```python
from build123d import *

# Parameters (mm, degrees)
SKETCH1_R           = 1.5
BOSS_EXTRUDE1_DEPTH = 5


with BuildPart() as part:
    # Sketch1 → Boss-Extrude1 (new body)
    with BuildSketch(Plane.XY):
        with BuildLine():
            Line((75.000000208, -15), (-75.000000208, -15))
            Line((-75.000000208, -15), (-75.000000208, 15))
            Line((-75.000000208, 15), (75.000000208, 15))
            ThreePointArc((75.000000208, 15), (89.999999792, 0), (75.000000208, -15))
        make_face()
        with Locations((75, 7)):
            Circle(SKETCH1_R, mode=Mode.SUBTRACT)
        with Locations((82, 0)):
            Circle(SKETCH1_R, mode=Mode.SUBTRACT)
        with Locations(Location((68, 0, 0), (0, 0, 180))):
            Circle(SKETCH1_R, mode=Mode.SUBTRACT)
        with Locations(Location((75, -7, 0), (0, 0, 180))):
            Circle(SKETCH1_R, mode=Mode.SUBTRACT)
        with Locations((-63.000000208, 0)):
            Circle(SKETCH1_R, mode=Mode.SUBTRACT)
        with Locations((-63.000000208, 10)):
            Circle(SKETCH1_R, mode=Mode.SUBTRACT)
        with Locations((-63.000000208, -10)):
            Circle(SKETCH1_R, mode=Mode.SUBTRACT)
    extrude(amount=BOSS_EXTRUDE1_DEPTH)


solid = part.part
```
Model file for the job. Use its own axes, mm. Give positions to 0.01 mm unless a question says otherwise; leave off trailing zeros. Loops run counter-clockwise (first coordinate to the right, second up) from the corner with the lowest first, then second, coordinate; pieces in that order, holes last. Notation, with made-up numbers: (47.25, 22.25) - (65.25, 22.25) arc R8 ccw to (65.25, 36.25) - close; hole circle Ø4 at (6.5, 63.5). An arc over 180 degrees is marked (long way). One line per item, written item: value. Start each with the question number.
1. Slice it at A-A (y = 0). List the corners of the cut face in (x, z).
2. Slice it at B-B (z = 1.55). List the corners of the cut face in (x, y).
3. Slice it at D-D (x = -63). List the corners of the cut face in (y, z).
4. Slice it at C-C (x = 68). List the corners of the cut face in (y, z).
5. Pull direction Y, two halves, no side cores. Call faces 1 (the flat face through (-1, 15, 2)), 2 (the cylindrical face through (-64.2, 9.1, 2.5)), 3 (the flat face through (9, 0, 5)): pulls with the +Y half, pulls with the -Y half, needs draft (parallel to the pull), parting line crosses it, or undercut.
6. Probe L1, parallel to Y at x = -63, z = 2.3; L2, parallel to X at y = 9, z = 1.5; L3, parallel to Y at x = 82, z = 4. List the from-to ranges inside material, lowest first. Write a range as from..to.
Solution:
1. outline: (-75, 0) - (-64.5, 0) - (-64.5, 5) - (-75, 5) - close; (-61.5, 0) - (66.5, 0) - (66.5, 5) - (-61.5, 5) - close; (69.5, 0) - (80.5, 0) - (80.5, 5) - (69.5, 5) - close; (83.5, 0) - (90, 0) - (90, 5) - (83.5, 5) - close
2. outline: (-75, -15) - (75, -15) arc R15 ccw to (75, 15) - (-75, 15) - close; hole circle Ø3 at (-63, -10); hole circle Ø3 at (-63, 0); hole circle Ø3 at (-63, 10); hole circle Ø3 at (68, 0); hole circle Ø3 at (75, -7); hole circle Ø3 at (75, 7); hole circle Ø3 at (82, 0)
3. outline: (-15, 0) - (-11.5, 0) - (-11.5, 5) - (-15, 5) - close; (-8.5, 0) - (-1.5, 0) - (-1.5, 5) - (-8.5, 5) - close; (1.5, 0) - (8.5, 0) - (8.5, 5) - (1.5, 5) - close; (11.5, 0) - (15, 0) - (15, 5) - (11.5, 5) - close
4. outline: (-15, 0) - (-1.5, 0) - (-1.5, 5) - (-15, 5) - close; (1.5, 0) - (15, 0) - (15, 5) - (1.5, 5) - close
5. face 1: pulls with the +Y half
5. face 2: undercut
5. face 3: needs draft
6. L1: y = -15..-11.5, -8.5..-1.5, 1.5..8.5, 11.5..15
6. L2: x = -75..-64.12, -61.88..87
6. L3: y = -13.27..-1.5, 1.5..13.27
